```python
from build123d import *

# Parameters (mm, degrees)
BOSS_EXTRUDE1_DEPTH = 7
SKETCH2_R           = 7.5
BOSS_EXTRUDE2_DEPTH = 2


with BuildPart() as part:
    # Sketch1 → Boss-Extrude1 (new body)
    with BuildSketch(Plane(origin=(0, 0, 0), x_dir=(1, 0, 0), z_dir=(0, 1, 0))):
        Polygon((-15.307337295, -36.9551813), (-5.96952274, 1.939615515), (5.96952274, 1.939615515), (15.307337295, -36.9551813), (0.906459551, -2.188386941), (-0.906459551, -2.188386941), align=None)
    extrude(amount=BOSS_EXTRUDE1_DEPTH)

    # Sketch2 → Boss-Extrude2 (add)
    with BuildSketch(Plane(origin=(0, 0, -1.939615515), x_dir=(-1, 0, 0), z_dir=(0, 0, -1))):
        with Locations((0, 3.5)):
            Circle(SKETCH2_R)
    extrude(amount=BOSS_EXTRUDE2_DEPTH)


solid = part.part
```
Model file for the job. Use its own axes, mm. A direction names the side the tool comes from. Give positions to 0.01 mm unless a question says otherwise; leave off trailing zeros. Write each loop counter-clockwise with the first axis right and the second up, starting at its lowest first coordinate (ties: lowest second). Pieces come first, ordered by that corner, then holes. Notation, with made-up numbers: (-18, 72.5) - (27, 72.5) arc R18 cw to (27, 89.5) - close; hole circle Ø8 at (23.5, 54). An arc over 180 degrees is marked (long way). One line per question, with ' | ' between items. Start each with the question number.
(1) Slice it at D-D on x = 11.5. Write the cut outline in (y, z).
(2) Slice it at A-A on y = 3.5. Write the cut outline in (x, z).
(3) Pin check, flat tips, straight feed: P1, Ø2, axis at x = -9, z = 21.5, coming from the -Y side; P2, Ø1.5, axis at y = 4, z = 6, coming from the -X side; P3, Ø8, axis at x = -10, y = 1, coming from the +Z side. Stop position of each tip, or through.
(4) 3-axis set-ups, long thin cutter, end or side, ignore diameter. For faces 4 (the face through (0, 3, 2.188)), 5 (the face through (10.573, 3.451, 17.236)), 6 (the face through (-4.5, 0, 10.2)), 7 (the face through (0.976, 10.936, -2.926)): which of +Z, -Z, +X, -X, +Y, -Y reach the whole face in a straight line?
(5) Wall check: line 1 along Y through (x, z) = (-4, 1); line 2 along X through (y, z) = (4.25, 26); line 3 along X through (y, z) = (4.5, 6). Give the ranges that are in metal, low to high. Write a range as from..to.
(6) Slice it at B-B on x = 0. Write the cut outline in (y, z).
(7) Slice it at C-C on y = 1.25. Write the cut outline in (x, z).
(8) Two-plate mould, pull along X, no slides. Class faces 1 (the face through (-8.006, 3.451, 19.328)), 2 (the face through (-4.5, 7, 10.2)), 3 (the face through (-10.704, 3.451, 17.78)): +X half, -X half, draft (parallel to the pull), parting line (faces both ways), or undercut.
Results below:
1) outline: (0, 21.1) - (7, 21.1) - (7, 27.76) - (0, 27.76) - close
2) outline: (-15.31, 36.96) - (-5.97, -1.94) - (-7.5, -1.94) - (-7.5, -3.94) - (7.5, -3.94) - (7.5, -1.94) - (5.97, -1.94) - (15.31, 36.96) - (0.91, 2.19) - (-0.91, 2.19) - close
3) P1: y = 0 | P2: x = -8.06 | P3: z = 33.8
4) face 4: +Z, +Y, -Y | face 5: +X, +Y, -Y | face 6: +Z, +X, -X, -Y | face 7: -Z
5) line 1: 0..7 | line 2: -12.68..-10.77, 10.77..12.68 | line 3: -7.88..-2.49, 2.49..7.88
6) outline: (-4, -3.94) - (11, -3.94) - (11, -1.94) - (7, -1.94) - (7, 2.19) - (0, 2.19) - (0, -1.94) - (-4, -1.94) - close
7) outline: (-15.31, 36.96) - (-5.97, -1.94) - (-7.15, -1.94) - (-7.15, -3.94) - (7.15, -3.94) - (7.15, -1.94) - (5.97, -1.94) - (15.31, 36.96) - (0.91, 2.19) - (-0.91, 2.19) - close
8) face 1: undercut | face 2: draft | face 3: -X half
